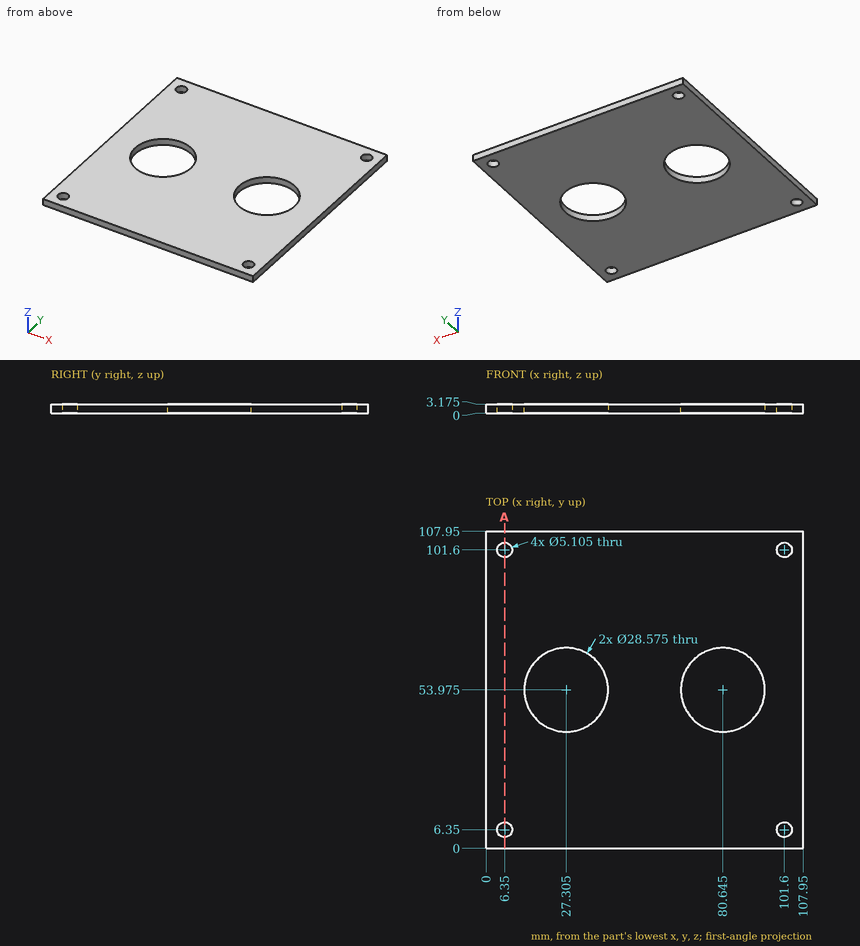
Can you work these out from the drawing? Everything is in mm from the part's minimum corner. Round coordinates to 2 decimals unless told otherwise and drop trailing zeros. One line per question, with ' | ' between items. Start each with the question number.
Q1. Will these pins go through, and if not, where does the flat tip stop? pin 1 (4.5 mm diameter, centred on x = 101.6, y = 6.35, fed in from +Z); pin 2 (6 mm diameter, centred on x = 101.6, y = 101.6, fed in from +Z) (3 decimals).
Q2. I want a section at A-A (x = 6.35). State how many separate pieces and enclosed holes the cut face has, then the cut area to 3 significant figures.
Q3. Please list where these lines run through material, in increasing order: line 1 (Y direction, x = 6.35, z = 2.55); line 2 (X direction, y = 63, z = 2.9); line 3 (X direction, y = 41.5, z = 1.95). Write a range as [from, to].
Response values:
1) pin 1: passes through | pin 2: stops at z = 3.175
2) separate pieces: 3 | enclosed holes: 0 | area: 310 mm²
3) line 1: y = [0, 3.8], [8.9, 99.05], [104.15, 107.95] | line 2: x = [0, 16.23], [38.38, 69.57], [91.72, 107.95] | line 3: x = [0, 20.34], [34.27, 73.68], [87.61, 107.95]
